For this review, take the finished solid that the model builds, in its own axes (mm). A direction names the side the tool comes from. Give positions to 0.01 mm unless a question says otherwise; leave off trailing zeros. Loops run counter-clockwise (first coordinate to the right, second up) from the corner with the lowest first, then second, coordinate; pieces in that order, holes last.
```python
from build123d import *

# Parameters (mm, degrees)
CUT_EXTRUDE_1_DEPTH      = 120.272796563
CUT_EXTRUDE_1_DEPTH_BACK = 120.272796563
SKETCH_2_W               = 6
SKETCH_2_H               = 4
SKETCH_2_W_2             = 6.5
SKETCH_2_H_2             = 15


with BuildPart() as part:
    # Эскиз1 → Повернуть1 (revolve)
    with BuildSketch(Plane.XY, mode=Mode.PRIVATE) as revolve_1_sk:
        Polygon((0, 39), (6, 39), (6, 35.5), (51, 35.5), (51, 40.5), (54, 40.5), (54, 40), (75, 40), (76, 41), (76, 47.5), (58.679491924, 57.5), (9, 57.5), (9, 57), (6, 57), (6, 65), (0, 65), align=None)
    revolve(revolve_1_sk.sketch.rotate(Axis((0, 0, 0), (1, 0, 0)), 90), axis=Axis((0, 0, 0), (1, 0, 0)))

    # Эскиз2 → Вырез-Вытянуть1 (cut, two sides: drawn at the far end of the back side and taken through both)
    with BuildSketch(Plane.XY.offset(-CUT_EXTRUDE_1_DEPTH_BACK)):
        with Locations((45, 55.5)):
            Rectangle(SKETCH_2_W, SKETCH_2_H)
        with Locations((3.25, 0)):
            Rectangle(SKETCH_2_W_2, SKETCH_2_H_2)
    extrude(amount=CUT_EXTRUDE_1_DEPTH + CUT_EXTRUDE_1_DEPTH_BACK, mode=Mode.SUBTRACT)


solid = part.part
```
Item 1: Clearance check with flat-ended pins moving along their axes: pin 1 Ø10 at (x, y) = (20.5, 40) entering from -Z; pin 2 Ø2 at (x, z) = (2.5, 53.5) entering from -Y; pin 3 Ø2 at (x, z) = (2, 51) entering from +Y; pin 4 Ø25 at (y, z) = (16, -14) entering from -X. State where each tip first meets the part, or that it passes through.
Answer:
pin 1: stops at z = -45.62
pin 2: stops at y = -38.32
pin 3: stops at y = 41.53
pin 4: passes through
Item 2: Tool access review of faces 1 (the flat face through (51, 36, 0)), 2 (the cylindrical face through (2.958, -64.987, 1.324)), 3 (the flat face through (6.5, 0, 46)), 4 (the cylindrical face through (3.042, -38.993, 0.752)), 5 (the flat face through (42, 55, 0)): name each direction out of +Z, -Z, +X, -X, +Y, -Y from which nothing blocks a thin tool from reaching the whole face with its end or side.
Answer:
face 1: none
face 2: +X, -X, -Y
face 3: +Z, -Z, -X
face 4: -X
face 5: +Z, -Z, +Y
Item 3: Take a section at B-B on x = 36. Give the boundary of the cut face in (y, z).
Answer:
outline: circle Ø115 at (0, 0); hole circle Ø71 at (0, 0)
Item 4: For L1, parallel to Z at x = 24.5, y = 0.5; L2, parallel to Y at x = 53.4, z = 0, list the stretches that pass through material, from the lowest coordinate up.
Answer:
L1: z = -57.5 to -35.5, 35.5 to 57.5
L2: y = -57.5 to -40.5, 40.5 to 57.5
Item 5: Take a section at A-A on y = 0. Give the boundary of the cut face in (x, z), and give its area (3 significant figures).
Answer:
outline: (6.5, -57) - (9, -57) - (9, -57.5) - (58.68, -57.5) - (76, -47.5) - (76, -41) - (75, -40) - (54, -40) - (54, -40.5) - (51, -40.5) - (51, -35.5) - (6.5, -35.5) - close; (6.5, 35.5) - (51, 35.5) - (51, 40.5) - (54, 40.5) - (54, 40) - (75, 40) - (76, 41) - (76, 47.5) - (58.68, 57.5) - (9, 57.5) - (9, 57) - (6.5, 57) - close
area: 2,650 mm2
Item 6: The part is to be moulded in two halves that separate along Z. For faces 6 (the cylindrical face through (52.521, -40.155, -5.272)), 7 (the conical face through (74.9, 47, -10.4)), 8 (the flat face through (0, -43, -1)), say which applies: released by +Z, released by -Z, zero draft, split by the parting line, or undercut.
Answer:
face 6: undercut
face 7: split by the parting line
face 8: zero draft
